from build123d import *

# Parameters (mm, degrees)
F0_R     = 22.225
F1_DEPTH = 12.7
F0_R_2   = 14.2875
F0_R_3   = 9.525
F2_DEPTH = 22.225


with BuildPart() as f1:
    # F0 (on Front) → F1 (new body, symmetric)
    with BuildSketch(Plane.XZ):
        with BuildLine():
            ThreePointArc((0.971786, 52.628446), (1.432993, 50.145594), (1.5875, 47.625))
            ThreePointArc((1.5875, 47.625), (-19.05, 26.9875), (-39.6875, 47.625))
            ThreePointArc((-39.6875, 47.625), (-53.837568, 28.249011), (-75.9968, 19.05))
            Line((-75.9968, 19.05), (-63.2968, 19.05))
            ThreePointArc((-63.2968, 19.05), (-44.2468, 0), (-63.2968, -19.05))
            Line((-63.2968, -19.05), (-88.6968, -19.05))
            Line((-88.6968, -19.05), (-8.395337, -37.002993))
            ThreePointArc((-8.395337, -37.002993), (12.439533, -35.863776), (29.616348, -24.016978))
            ThreePointArc((29.616348, -24.016978), (38.533005, -18.624111), (48.872514, -19.921925))
            ThreePointArc((48.872514, -19.921925), (70.450489, -18.880117), (80.9498, 0))
            ThreePointArc((80.9498, 0), (76.233903, 27.779937), (62.281711, 52.26056))
            ThreePointArc((62.281711, 52.26056), (44.883221, 57.23725), (29.550918, 47.625))
            ThreePointArc((29.550918, 47.625), (13.635509, 40.840087), (0.971786, 52.628446))
        make_face()
        Circle(F0_R, mode=Mode.SUBTRACT)
        with BuildLine():
            ThreePointArc((69.85, 0), (58.7248, -11.1252), (47.5996, 0))
            ThreePointArc((47.5996, 0), (44.728993, 16.280022), (36.463409, 30.596433))
            ThreePointArc((36.463409, 30.596433), (37.92717, 46.15973), (53.508204, 44.898715))
            ThreePointArc((53.508204, 44.898715), (65.63753, 23.890107), (69.85, 0))
        make_face(mode=Mode.SUBTRACT)
    extrude(amount=F1_DEPTH, both=True)

    # F0 (on Front) → F2 (join, symmetric)
    with BuildSketch(Plane.XZ):
        Circle(F0_R)
        Circle(F0_R_2, mode=Mode.SUBTRACT)
        with BuildLine():
            Line((-63.2968, 19.05), (-75.9968, 19.05))
            Line((-75.9968, 19.05), (-88.6968, 19.05))
            ThreePointArc((-88.6968, 19.05), (-107.7468, 0), (-88.6968, -19.05))
            Line((-88.6968, -19.05), (-63.2968, -19.05))
            ThreePointArc((-63.2968, -19.05), (-44.2468, 0), (-63.2968, 19.05))
        make_face()
        with BuildLine():
            ThreePointArc((-88.6968, -11.0998), (-99.7966, 0), (-88.6968, 11.0998))
            Line((-88.6968, 11.0998), (-63.2968, 11.0998))
            ThreePointArc((-63.2968, 11.0998), (-52.197, 0), (-63.2968, -11.0998))
            Line((-63.2968, -11.0998), (-88.6968, -11.0998))
        make_face(mode=Mode.SUBTRACT)
        with BuildLine():
            ThreePointArc((-39.6875, 47.625), (-19.05, 26.9875), (1.5875, 47.625))
            ThreePointArc((1.5875, 47.625), (1.432993, 50.145594), (0.971786, 52.628446))
            ThreePointArc((0.971786, 52.628446), (-21.570594, 68.107993), (-39.6875, 47.625))
        make_face()
        with Locations((-19.05, 47.625)):
            Circle(F0_R_3, mode=Mode.SUBTRACT)
    extrude(amount=F2_DEPTH, both=True)


solid = f1.part
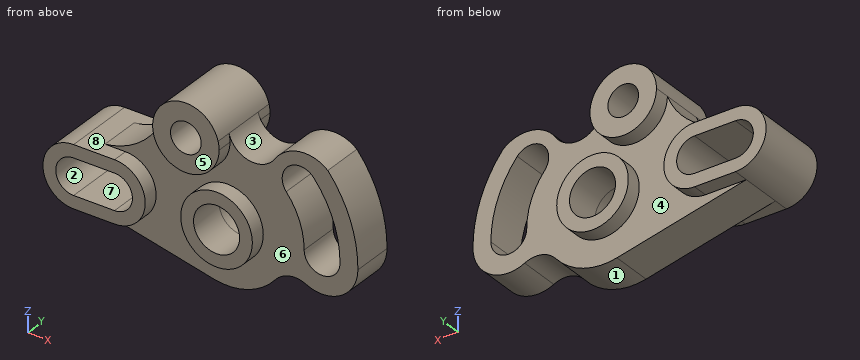
Input: part model. Units: mm. Frame: model coordinates. Face numbers are marked on the shaded views. A direction names the side the tool comes from. Give positions to 0.01 mm unless a question says otherwise; leave off trailing zeros. Order: outer loops, then holes, each group sorted by start corner. A loop starts at its lowest first (then second) coordinate and runs counter-clockwise, first axis right, second up. Notation, with made-up numbers: (76, 19) -> (120, 19) arc R24 cw to (120, 49) -> close; hole circle Ø10 at (-18.5, -34). An arc over 180 degrees is marked (long way). Use one line per item in the form item = value.
1) Line query: probe 1 along X at (y, z) = (4, -0.5); probe 2 along X at (y, z) = (-3, 11.5); probe 3 along X at (y, z) = (-17.5, -12). Output: solid intervals per line, ascending.
Response values:
probe_1 = -107.74 to -99.79, -52.21 to -14.28, 14.28 to 47.61, 69.84 to 80.94
probe_2 = -103.88 to -8.48, 8.48 to 46.19, 68.9 to 80.21
probe_3 = -103.49 to -48.5, -18.71 to -7.75, 7.75 to 18.71
2) First-contact query: pin 1 Ø7.5 at (x, y) = (-76.5, -0.5) entering from +Z; pin 2 Ø17 at (x, z) = (0, 0) entering from +Y; pin 3 Ø8 at (y, z) = (16.5, 2) entering from -X; pin 4 Ø1 at (x, y) = (50.5, 2) entering from -Z. Flat tips, straight axial feed; report the tip coordinate or a pass-through.
Response values:
pin_1 = 19.56
pin_2 = through
pin_3 = -107.75
pin_4 = -20.84
3) Section C-C, the plane x = 6.5. Return loops of the section in (y, z) (3 decimals).
Response values:
outline = (-22.225, -21.253) -> (-12.7, -21.253) -> (-12.7, -37.377) -> (12.7, -37.377) -> (12.7, -21.253) -> (22.225, -21.253) -> (22.225, -12.723) -> (-22.225, -12.723) -> close; (-22.225, 12.723) -> (22.225, 12.723) -> (22.225, 21.253) -> (12.7, 21.253) -> (12.7, 44.046) -> (-12.7, 44.046) -> (-12.7, 21.253) -> (-22.225, 21.253) -> close
4) Section A-A, the plane x = -73.5. Return loops of the section in (y, z) (3 decimals).
Response values:
outline = (-22.225, -19.05) -> (-12.7, -19.05) -> (-12.7, -22.448) -> (12.7, -22.448) -> (12.7, -19.05) -> (22.225, -19.05) -> (22.225, -11.1) -> (-22.225, -11.1) -> close; (-22.225, 11.1) -> (22.225, 11.1) -> (22.225, 19.05) -> (12.7, 19.05) -> (12.7, 19.424) -> (-12.7, 19.424) -> (-12.7, 19.05) -> (-22.225, 19.05) -> close
5) Mould query, pull axis Z, two halves, no side actions, for the marked faces 1, 2 and 3. Classes: pulls with the +Z half, pulls with the -Z half, needs draft (parallel to the pull), parting line crosses it, or undercut.
Response values:
face_1 = pulls with the -Z half
face_2 = undercut
face_3 = pulls with the +Z half
6) Reachability of the marked faces 4, 5, 6, 7 and 8 from +Z, -Z, +X, -X, +Y, -Y: full face, straight path, thin tool, end or side. Return the list, or none.
Response values:
face_4 = +Y
face_5 = +Z, -Z, +X, -X, -Y
face_6 = -Y
face_7 = +Y, -Y
face_8 = +Z, -X
7) Section D-D, the plane z = 60. Return loops of the section in (x, y) (3 decimals), and give its area (3 significant figures).
Response values:
outline = (-35.566, -22.225) -> (-2.534, -22.225) -> (-2.534, 22.225) -> (-35.566, 22.225) -> close
area = 1,470 mm^2
8) Section B-B, the plane y = -2.5. Count the separate pieces of the cut face and the enclosed holes in it, and give its area (3 significant figures).
Response values:
separate_pieces = 1
enclosed_holes = 4
area = 9,500 mm^2
